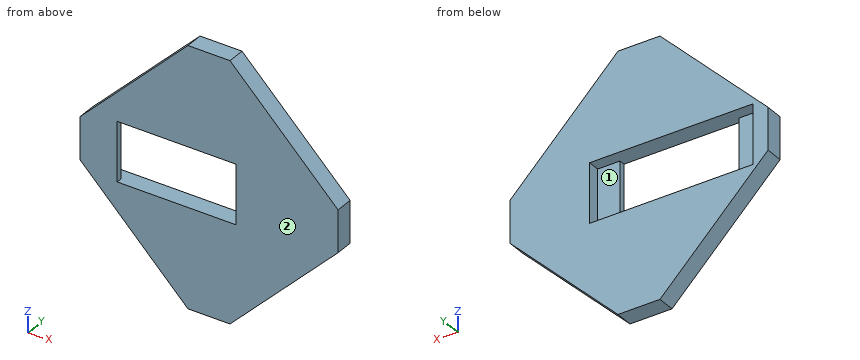
```python
from build123d import *

# Parameters (mm, degrees)
BOSS_EXTRUDE1_DEPTH = 6
SKETCH1_3_W         = 7.5
SKETCH1_3_H         = 20
BOSS_EXTRUDE2_DEPTH = 2


with BuildPart() as part:
    # Sketch1 → Boss-Extrude1 (new body)
    with BuildSketch(Plane(origin=(0, 0, 0), x_dir=(1, 0, 0), z_dir=(0, 1, 0))):
        Polygon((43.450252532, 7.071067812), (7.071067812, 43.450252532), (-7.071067812, 43.450252532), (-43.450252532, 7.071067812), (-43.450252532, -7.071067812), (-7.071067812, -43.450252532), (7.071067812, -43.450252532), (43.450252532, -7.071067812), align=None)
        Polygon((-30.9, -10), (-38.4, -10), (-38.4, 10), (-30.9, 10), (9.1, 10), (16.6, 10), (16.6, -10), (9.1, -10), align=None, mode=Mode.SUBTRACT)
    extrude(amount=BOSS_EXTRUDE1_DEPTH)

    # Sketch1<3> → Boss-Extrude2 (add)
    with BuildSketch(Plane(origin=(0, 0, 0), x_dir=(1, 0, 0), z_dir=(0, 1, 0))):
        with Locations((-34.65, 0)):
            Rectangle(SKETCH1_3_W, SKETCH1_3_H)
        with Locations((12.85, 0)):
            Rectangle(SKETCH1_3_W, SKETCH1_3_H)
    extrude(amount=BOSS_EXTRUDE2_DEPTH)


solid = part.part
```
Build history of the part. All positions in model axes, mm. Face numbers are marked on the shaded views. Coordinates: 2 decimals unless noted, no trailing zeros. Order: outer loops, then holes, each group sorted by start corner. A loop starts at its lowest first (then second) coordinate and runs counter-clockwise, first axis right, second up.
Item 1: Drop flat-ended pins along their axis: pin 1 Ø6 at (x, z) = (12, 4.5) entering from +Y; pin 2 Ø1.5 at (x, y) = (-10.5, 2.5) entering from -Z; pin 3 Ø1.5 at (y, z) = (0.5, 15.5) entering from -X. Give the stop position or say it passes through.
Filled in:
pin 1: stops at y = 2
pin 2: stops at z = -40.77
pin 3: stops at x = -35.77
Item 2: Saw through at B-B on z = 9. List the corners of the cut face in (x, y), then the cut area to 3 significant figures.
Filled in:
outline: (-41.52, 0) - (-30.9, 0) - (-30.9, 2) - (-38.4, 2) - (-38.4, 6) - (-41.52, 6) - close; (9.1, 0) - (41.52, 0) - (41.52, 6) - (16.6, 6) - (16.6, 2) - (9.1, 2) - close
area: 198 mm2
Item 3: Drill centre lines: L1, parallel to Z at x = -2.5, y = 5.4; L2, parallel to X at y = 2.9, z = -1; L3, parallel to X at y = 2.3, z = 9.5. Where is each one in solid material? Low to high.
Filled in:
L1: z = -43.45 to -10, 10 to 43.45
L2: x = -43.45 to -38.4, 16.6 to 43.45
L3: x = -41.02 to -38.4, 16.6 to 41.02
Item 4: Saw through at C-C on x = -27. List the corners of the cut face in (y, z), then the cut area to 3 significant figures.
Filled in:
outline: (0, -23.52) - (6, -23.52) - (6, -10) - (0, -10) - close; (0, 10) - (6, 10) - (6, 23.52) - (0, 23.52) - close
area: 162 mm2
Item 5: Mould opens along Z. For the marked faces 1 and 2 say: released by +Z, released by -Z, zero draft, split by the parting line, or undercut.
Filled in:
face 1: undercut
face 2: zero draft
Item 6: Saw through at D-D on z = -5. List the corners of the cut face in (x, y), then the cut area to 3 significant figures.
Filled in:
outline: (-43.45, 0) - (-30.9, 0) - (-30.9, 2) - (-38.4, 2) - (-38.4, 6) - (-43.45, 6) - close; (9.1, 0) - (43.45, 0) - (43.45, 6) - (16.6, 6) - (16.6, 2) - (9.1, 2) - close
area: 221 mm2
Item 7: Saw through at A-A on y = 1.1. List the corners of the cut face in (x, z), then the cut area to 3 significant figures.
Filled in:
outline: (-43.45, -7.07) - (-7.07, -43.45) - (7.07, -43.45) - (43.45, -7.07) - (43.45, 7.07) - (7.07, 43.45) - (-7.07, 43.45) - (-43.45, 7.07) - close; hole (-30.9, -10) - (9.1, -10) - (9.1, 10) - (-30.9, 10) - close
area: 4,100 mm2
